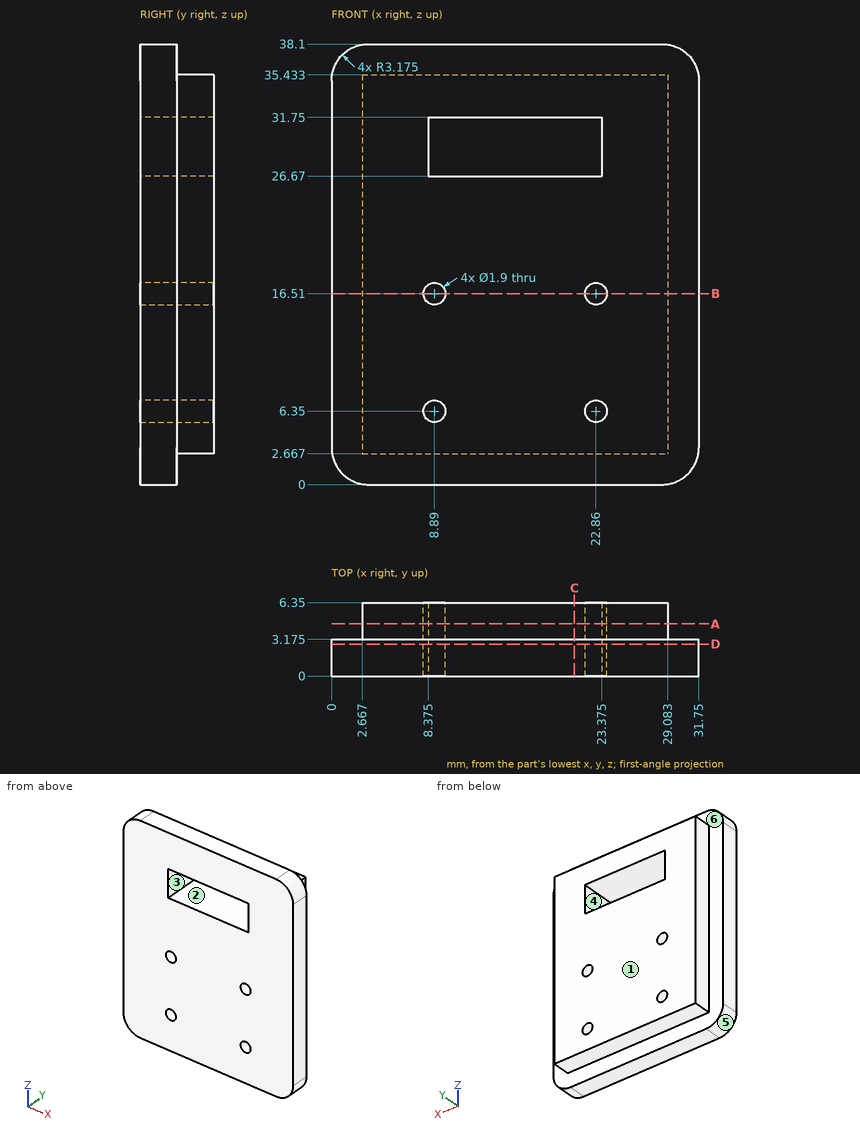
Source: three-view drawing plus pictorial views. Frame: mm from the lowest corner of the part. A direction names the side the tool comes from. Coordinates: 2 decimals unless noted, no trailing zeros. Loops run counter-clockwise (first coordinate to the right, second up) from the corner with the lowest first, then second, coordinate; pieces in that order, holes last. Notation, with made-up numbers: (77, -30) - (109, -30) arc R24 ccw to (109, -20) - close; hole circle Ø1 at (41.25, -2.5). An arc over 180 degrees is marked (long way). One line per item, written item: value. Start each with the question number.
1. Section B-B (z = 16.51). Return the cut outline in (x, y) (3 decimals), and give its area (3 significant figures).
2. Section C-C (x = 21). Return the cut outline in (y, z) (3 decimals).
3. Section A-A (y = 4.5). Return the cut outline in (x, z) (3 decimals).
4. Mould query, pull axis X, two halves, no side actions, for the marked faces 3, 4, 5 and 6. Classes: pulls with the +X half, pulls with the -X half, needs draft (parallel to the pull), parting line crosses it, or undercut.
5. Set-up query: the marked faces 1 and 2. Return all of +Z, -Z, +X, -X, +Y, -Y with unobstructed straight access to the full face (end or side cutting, diameter ignored); none if empty.
6. Section D-D (y = 2.75). Return the cut outline in (x, z) (3 decimals).
7. Ray query, L1, parallel to X at y = 3.25, z = 16.51; L2, parallel to X at y = 2.25, z = 16.51; L3, parallel to Z at x = 23, y = 4.5. Return the intervals inside material, ascending.
8. Contact query for flat-ended pins moving along their axis: P1, Ø3.5, axis at x = 14, y = 5, coming from the +Z side; P2, Ø1, axis at x = 20, y = 5, coming from the -Z side; P3, Ø2.5, axis at y = 4.5, z = 21, coming from the +X side. Output: stop coordinate, or through.
Verdict:
1. outline: (0, 0) - (7.94, 0) - (7.94, 6.35) - (2.667, 6.35) - (2.667, 3.175) - (0, 3.175) - close; (9.84, 0) - (21.91, 0) - (21.91, 6.35) - (9.84, 6.35) - close; (23.81, 0) - (31.75, 0) - (31.75, 3.175) - (29.083, 3.175) - (29.083, 6.35) - (23.81, 6.35) - close
1. area: 161 mm2
2. outline: (0, 0) - (3.175, 0) - (3.175, 2.667) - (6.35, 2.667) - (6.35, 26.67) - (0, 26.67) - close; (0, 31.75) - (6.35, 31.75) - (6.35, 35.433) - (3.175, 35.433) - (3.175, 38.1) - (0, 38.1) - close
3. outline: (2.667, 2.667) - (29.083, 2.667) - (29.083, 35.433) - (2.667, 35.433) - close; hole circle Ø1.9 at (8.89, 6.35); hole circle Ø1.9 at (8.89, 16.51); hole (8.375, 26.67) - (23.375, 26.67) - (23.375, 31.75) - (8.375, 31.75) - close; hole circle Ø1.9 at (22.86, 6.35); hole circle Ø1.9 at (22.86, 16.51)
4. face 3: undercut
4. face 4: undercut
4. face 5: pulls with the -X half
4. face 6: needs draft
5. face 1: +Z, -Z, +X, -X, +Y
5. face 2: +Y, -Y
6. outline: (0, 3.175) arc R3.175 ccw to (3.175, 0) - (28.575, 0) arc R3.175 ccw to (31.75, 3.175) - (31.75, 34.925) arc R3.175 ccw to (28.575, 38.1) - (3.175, 38.1) arc R3.175 ccw to (0, 34.925) - close; hole circle Ø1.9 at (8.89, 6.35); hole circle Ø1.9 at (8.89, 16.51); hole (8.375, 26.67) - (23.375, 26.67) - (23.375, 31.75) - (8.375, 31.75) - close; hole circle Ø1.9 at (22.86, 6.35); hole circle Ø1.9 at (22.86, 16.51)
7. L1: x = 2.67 to 7.94, 9.84 to 21.91, 23.81 to 29.08
7. L2: x = 0 to 7.94, 9.84 to 21.91, 23.81 to 31.75
7. L3: z = 2.67 to 5.41, 7.29 to 15.57, 17.45 to 26.67, 31.75 to 35.43
8. P1: stops at z = 35.43
8. P2: stops at z = 2.67
8. P3: stops at x = 29.08
